For this review, use the dimensioned drawing (mm, ordinates from the lowest corner) and the shaded views. Give positions to 0.01 mm unless a question says otherwise; leave off trailing zeros. Write each loop counter-clockwise with the first axis right and the second up, starting at its lowest first coordinate (ties: lowest second). Pieces come first, ordered by that corner, then holes.
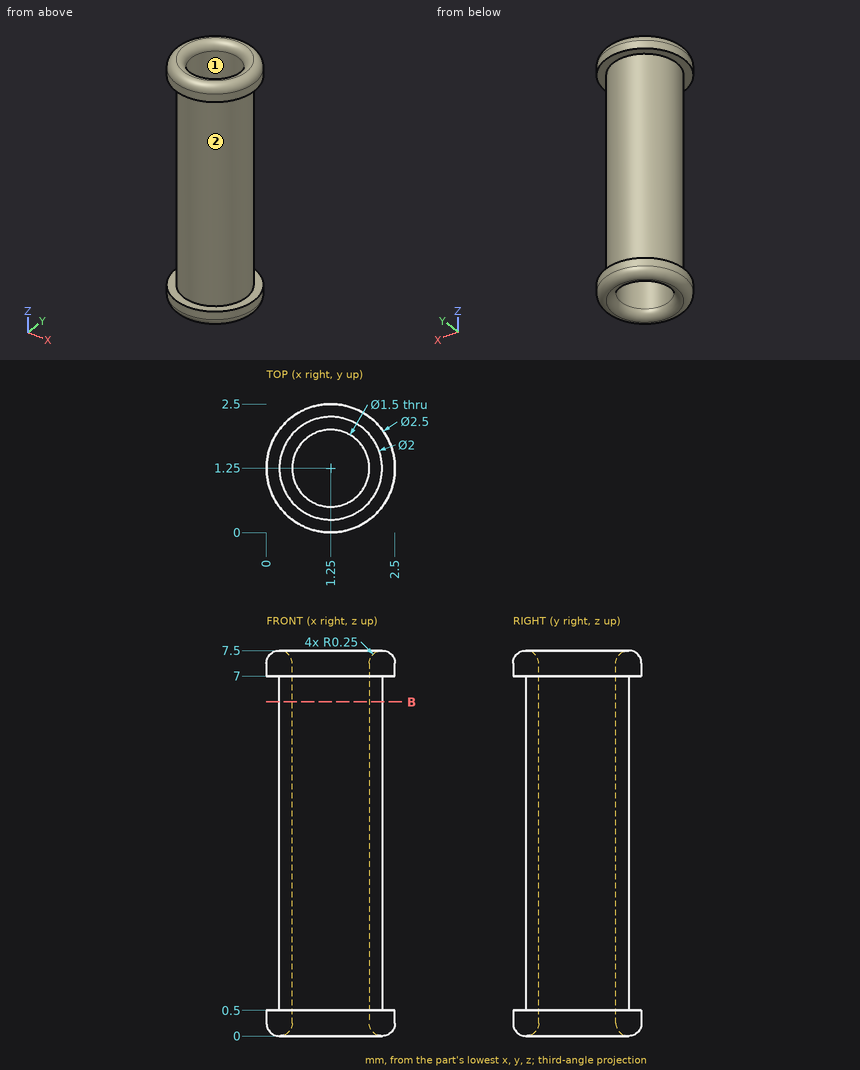
(1) For L1, parallel to Y at x = 1.25, z = 3.5; L2, parallel to X at y = 1.15, z = 6.75 (1 decimal); L3, parallel to Y at x = 0.9, z = 4, list the stretches that pass through material, from the lowest coordinate up.
(2) The part is to be moulded in two halves that separate along Z. For the marked faces 1 and 2, say which applies: +Z half, -Z half, draft (parallel to the pull), parting line (faces both ways), or undercut.
(3) We need section B-B (z = 6.5). Write out the cut boundary in (x, y).
(4) Clearance check with flat-ended pins moving along their axes: pin 1 Ø1 at (y, z) = (1, 6) entering from +X; pin 2 Ø0.9 at (x, y) = (1.25, 1.25) entering from -Z. State where each tip first meets the part, or that it passes through.
The answers:
1. L1: y = 0.25 to 0.5, 2 to 2.25
1. L2: x = 0.3 to 0.5, 2 to 2.2
1. L3: y = 0.31 to 0.59, 1.91 to 2.19
2. face 1: draft
2. face 2: undercut
3. outline: circle Ø2 at (1.25, 1.25); hole circle Ø1.5 at (1.25, 1.25)
4. pin 1: stops at x = 2.25
4. pin 2: passes through
